Read the model definition and answer for the solid it produces. Units are mm, in the model's axes. Face numbers are marked on the shaded views. A direction names the side the tool comes from. Coordinates: 2 decimals unless noted, no trailing zeros. Loops run counter-clockwise (first coordinate to the right, second up) from the corner with the lowest first, then second, coordinate; pieces in that order, holes last.
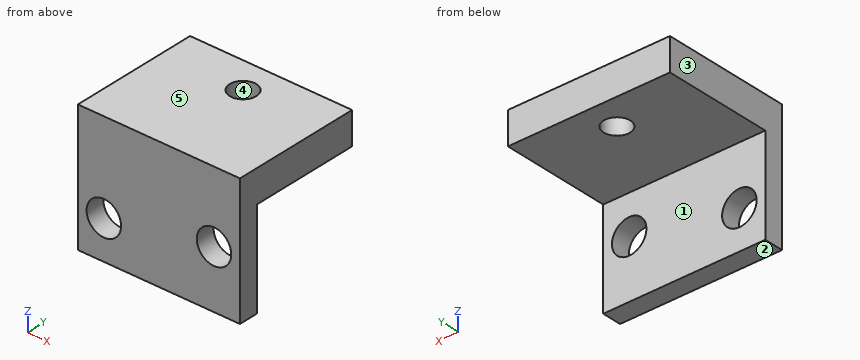
from build123d import *

# Parameters (mm, degrees)
BOSS_EXTRUDE1_DEPTH = 31.75
SKETCH3_R           = 2.6035
CUT_EXTRUDE1_DEPTH  = 45.901280605
SKETCH4_R           = 3.3782
CUT_EXTRUDE2_DEPTH  = 45.901280605
SKETCH5_W           = 31.75
SKETCH5_H           = 19.05
CUT_EXTRUDE3_DEPTH  = 2.54


with BuildPart() as part:
    # Sketch2 → Boss-Extrude1 (new body)
    with BuildSketch(Plane(origin=(0, 0, 0), x_dir=(0, 0, -1), z_dir=(1, 0, 0))):
        Polygon((0, 0), (25.4, 0), (25.4, 6.35), (6.35, 6.35), (6.35, 25.4), (0, 25.4), align=None)
    extrude(amount=BOSS_EXTRUDE1_DEPTH)

    # Sketch3 → Cut-Extrude1 (cut, through all)
    with BuildSketch(Plane(origin=(0, 0, -6.35), x_dir=(-1, 0, 0), z_dir=(0, 0, -1))):
        with Locations((-15.875, 19.05)):
            Circle(SKETCH3_R)
    extrude(amount=-CUT_EXTRUDE1_DEPTH, mode=Mode.SUBTRACT)

    # Sketch4 → Cut-Extrude2 (cut, through all)
    with BuildSketch(Plane(origin=(0, 6.35, 0), x_dir=(1, 0, 0), z_dir=(0, 1, 0))):
        with Locations(Location((5.08, 17.78, 0), (0, 0, 270))):
            Circle(SKETCH4_R)
        with Locations(Location((26.67, 13.97, 0), (0, 0, 270))):
            Circle(SKETCH4_R)
    extrude(amount=-CUT_EXTRUDE2_DEPTH, mode=Mode.SUBTRACT)

    # Sketch5 → Cut-Extrude3 (cut)
    with BuildSketch(Plane(origin=(0, 6.35, 0), x_dir=(1, 0, 0), z_dir=(0, 1, 0))):
        with Locations((15.875, 15.875)):
            Rectangle(SKETCH5_W, SKETCH5_H)
    extrude(amount=-CUT_EXTRUDE3_DEPTH, mode=Mode.SUBTRACT)


solid = part.part
Item 1: Find the intervals of material crossed by line 1 along X through (y, z) = (0.9, -13.97); line 2 along Z through (x, y) = (8.5, 10.25); line 3 along Y through (x, z) = (10, -12.5), in increasing order.
Numbers:
line 1: x = 0 to 23.29, 30.05 to 31.75
line 2: z = -6.35 to 0
line 3: y = 0 to 3.81
Item 2: Determine the mould class of the marked faces 3, 4 and 5 for opening direction X: released by +X, released by -X, zero draft, split by the parting line, or undercut.
Numbers:
face 3: released by -X
face 4: undercut
face 5: zero draft
Item 3: A cutting plane is placed at B-B on y = 19.05. Determine the outline of the cut face in (x, z).
Numbers:
outline: (0, -6.35) - (13.27, -6.35) - (13.27, 0) - (0, 0) - close; (18.48, -6.35) - (31.75, -6.35) - (31.75, 0) - (18.48, 0) - close
Item 4: A cutting plane is placed at D-D on x = 20. Determine the outline of the cut face in (y, z).
Numbers:
outline: (0, -25.4) - (3.81, -25.4) - (3.81, -6.35) - (25.4, -6.35) - (25.4, 0) - (0, 0) - close
Item 5: Which of the six approach directions +Z, -Z, +X, -X, +Y, -Y give full straight-line access (tool end or side, diameter ignored) to the marked faces 1 and 2?
Numbers:
face 1: -Z, +X, -X, +Y
face 2: -Z, +X, -X, +Y, -Y
Item 6: A cutting plane is placed at A-A on z = -13.97. Determine the outline of the cut face in (x, y), then the cut area to 3 significant figures.
Numbers:
outline: (0, 0) - (23.29, 0) - (23.29, 3.81) - (0, 3.81) - close; (30.05, 0) - (31.75, 0) - (31.75, 3.81) - (30.05, 3.81) - close
area: 95.2 mm2
Item 7: Given pin 1 (6 mm diameter, centred on x = 25, z = -21.5, fed in from +Y); pin 2 (6.5 mm diameter, centred on x = 8.5, y = 17.5, fed in from -Z), each flat-ended and moving along its own axis, determine where each tip first touches the part or whether it passes through.
Numbers:
pin 1: stops at y = 3.81
pin 2: stops at z = -6.35
Item 8: A cutting plane is placed at C-C on x = 6. Determine the outline of the cut face in (y, z), then the cut area to 3 significant figures.
Numbers:
outline: (0, -25.4) - (3.81, -25.4) - (3.81, -21.03) - (0, -21.03) - close; (0, -14.53) - (3.81, -14.53) - (3.81, -6.35) - (25.4, -6.35) - (25.4, 0) - (0, 0) - close
area: 209 mm2
